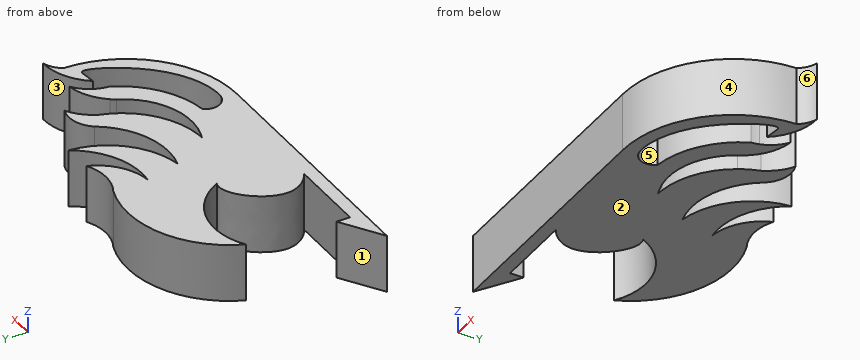
from build123d import *

# Parameters (mm, degrees)
F1_DEPTH = 25.4


with BuildPart() as f1:
    # F0 (on Top) → F1 (new body)
    with BuildSketch(Plane.XY):
        with BuildLine():
            add(Edge.make_bspline(
                [(-26.2610681984, -10.8273644), (-22.3250154222, -12.9399033802), (-6.7541943176, -14.1664240285), (-7.861061568, 17.5830890308), (-15.3270475566, 20.9516510367)],
                knots=[0.4911658302, 0.4911658302, 0.4911658302, 0.4911658302, 0.6402639099, 1, 1, 1, 1], degree=3))
            add(Edge.make_bspline(
                [(-15.3270475566, 20.9516510367), (-22.3564971203, 24.123253121), (-41.1418845104, 4.1977350509), (-30.2859655215, -8.6671412095), (-26.2610681984, -10.8273644)],
                knots=[0, 0, 0, 0, 0.3387023101, 0.4911658302, 0.4911658302, 0.4911658302, 0.4911658302], degree=3))
        make_face()
        with BuildLine():
            add(Edge.make_bspline(
                [(35.5182294418, -10.447258051), (31.9129186826, -10.220612291), (23.1955555043, -7.2820451281), (18.0529932429, 2.8715139484), (17.1729191086, 8.9899072036)],
                knots=[0.4660645619, 0.4660645619, 0.4660645619, 0.4660645619, 0.5346510085, 0.6442786993, 0.6442786993, 0.6442786993, 0.6442786993], degree=3))
            ThreePointArc((35.5182294418, -10.447258051), (30.0729748302, -6.5945561838), (31.0759395361, 0))
            ThreePointArc((31.0759395361, 0), (49.5151308357, 7.2590451113), (62.0112679899, 22.6390343159))
            ThreePointArc((62.0112679899, 22.6390343159), (62.2358256831, 24.395139963), (62.6415775007, 26.1184213282))
            add(Edge.make_bspline(
                [(54.4754700357, 26.7574300255), (57.3752815642, 26.5086516013), (60.1433747449, 26.2647226636), (62.6415775007, 26.1184213282)],
                knots=[0.9219128776, 0.9219128776, 0.9219128776, 0.9219128776, 0.9641346796, 0.9641346796, 0.9641346796, 0.9641346796], degree=3))
            ThreePointArc((54.4754700357, 26.7574300255), (53.7133787969, 25.7031684966), (53.0118979514, 24.6076434851))
            ThreePointArc((53.0118979514, 24.6076434851), (38.016967787, 10.0876095615), (17.1729191086, 8.9899072036))
        make_face()
        with BuildLine():
            ThreePointArc((-56.50515552, 32.3630547615), (-33.3182753375, 36.0316218628), (-15.3270475566, 20.9516510367))
            add(Edge.make_bspline(
                [(-26.2610681984, -10.8273644), (-22.3250154222, -12.9399033802), (-6.7541943176, -14.1664240285), (-7.861061568, 17.5830890308), (-15.3270475566, 20.9516510367)],
                knots=[0.4911658302, 0.4911658302, 0.4911658302, 0.4911658302, 0.6402639099, 1, 1, 1, 1], degree=3))
            Line((-26.2610681984, -10.8273644), (-60.464620338, -10.8273644))
            Line((-60.464620338, -10.8273644), (-60.464620338, -4.9215289764))
            Line((-60.464620338, -4.9215289764), (-78.4632340074, -16.4519678801))
            Line((-78.4632340074, -16.4519678801), (-14.9052012712, -16.4519678801))
            Line((-14.9052012712, -16.4519678801), (33.0445505679, -16.4519678801))
            ThreePointArc((33.0445505679, -16.4519678801), (67.0192612888, -2.5629170358), (81.5344079335, 31.1490573918))
            ThreePointArc((81.5344079335, 31.1490573918), (84.4106855525, 34.3353672495), (88.3062928915, 36.1380837858))
            ThreePointArc((88.3062928915, 36.1380837858), (77.0854781582, 33.5158631028), (68.3389529586, 26.0137952864))
            add(Edge.make_bspline(
                [(68.3389529586, 26.0137952864), (73.13500471, 26.2276507448), (80.3696253608, 30.0761350301), (65.6763095341, -1.3650666606), (43.6762193769, -10.9601053344), (35.5182294418, -10.447258051)],
                knots=[0, 0, 0, 0, 0.1043811632, 0.3108691907, 0.4660645619, 0.4660645619, 0.4660645619, 0.4660645619], degree=3))
            add(Edge.make_bspline(
                [(35.5182294418, -10.447258051), (31.9129186826, -10.220612291), (23.1955555043, -7.2820451281), (18.0529932429, 2.8715139484), (17.1729191086, 8.9899072036)],
                knots=[0.4660645619, 0.4660645619, 0.4660645619, 0.4660645619, 0.5346510085, 0.6442786993, 0.6442786993, 0.6442786993, 0.6442786993], degree=3))
            ThreePointArc((17.1729191086, 8.9899072036), (15.8161613784, 9.4543765839), (14.4833568484, 9.9836736917))
            ThreePointArc((14.4833568484, 9.9836736917), (15.7599932562, 10.0425488454), (17.0336540583, 10.1476914274))
            add(Edge.make_bspline(
                [(17.0336540583, 10.1476914274), (16.5524367293, 15.1345962527), (19.2361600934, 26.9166935874), (34.5605586177, 27.9160004318), (43.9602541666, 27.5027224979)],
                knots=[0.6512070875, 0.6512070875, 0.6512070875, 0.6512070875, 0.7409649976, 0.872432959, 0.872432959, 0.872432959, 0.872432959], degree=3))
            ThreePointArc((43.9602541666, 27.5027224979), (45.9259805238, 31.4321090753), (47.3872944713, 35.5756245553))
            ThreePointArc((47.3872944713, 35.5756245553), (51.1063153143, 41.2109006624), (56.3866607845, 45.4186797142))
            ThreePointArc((56.3866607845, 45.4186797142), (48.2264153253, 45.809802792), (41.481461376, 41.2002280354))
            ThreePointArc((41.481461376, 41.2002280354), (25.0576689955, 27.6740129875), (3.7966074888, 26.8574878573))
            ThreePointArc((3.7966074888, 26.8574878573), (23.5274065425, 37.3289516325), (32.4820913374, 57.7928125858))
            ThreePointArc((32.4820913374, 57.7928125858), (18.6619239349, 44.9253049217), (0, 42.0439206064))
            ThreePointArc((0, 42.0439206064), (12.1179065959, 46.7589869992), (19.8267325759, 57.2303533554))
            ThreePointArc((19.8267325759, 57.2303533554), (9.9133662879, 54.6642939776), (0, 57.2303533554))
            ThreePointArc((0, 57.2303533554), (-33.2620682112, 56.1796066262), (-56.50515552, 32.3630547615))
        make_face()
        with BuildLine():
            ThreePointArc((17.0336540583, 10.1476914274), (32.5838091219, 15.5874190212), (43.9602541666, 27.5027224979))
            add(Edge.make_bspline(
                [(17.0336540583, 10.1476914274), (16.5524367293, 15.1345962527), (19.2361600934, 26.9166935874), (34.5605586177, 27.9160004318), (43.9602541666, 27.5027224979)],
                knots=[0.6512070875, 0.6512070875, 0.6512070875, 0.6512070875, 0.7409649976, 0.872432959, 0.872432959, 0.872432959, 0.872432959], degree=3))
        make_face()
        with BuildLine():
            add(Edge.make_bspline(
                [(54.4754700357, 26.7574300255), (57.3752815642, 26.5086516013), (60.1433747449, 26.2647226636), (62.6415775007, 26.1184213282)],
                knots=[0.9219128776, 0.9219128776, 0.9219128776, 0.9219128776, 0.9641346796, 0.9641346796, 0.9641346796, 0.9641346796], degree=3))
            ThreePointArc((62.6415775007, 26.1184213282), (65.2892454144, 31.4686261622), (69.6213813016, 35.5756245553))
            ThreePointArc((69.6213813016, 35.5756245553), (61.1788209316, 32.6601387253), (54.4754700357, 26.7574300255))
        make_face()
    extrude(amount=F1_DEPTH)


solid = f1.part
Verification items for the finished model (mm, model axes). Face numbers are marked on the shaded views. A direction names the side the tool comes from. Coordinates: 2 decimals unless noted, no trailing zeros. Write each loop counter-clockwise with the first axis right and the second up, starting at its lowest first coordinate (ties: lowest second). Pieces come first, ordered by that corner, then holes. Notation, with made-up numbers: (85.25, 77.5) -> (103.25, 77.5) arc R20 ccw to (103.25, 96.5) -> close; hole circle Ø7 at (82, 12). An arc over 180 degrees is marked (long way). One line per item, written item: value. Start each with the question number.
Q1. Cross-section at C-C on y = 15. State how many separate pieces and enclosed holes the cut face has, and give its area (3 significant figures).
Q2. Access from +Z, -Z, +X, -X, +Y, -Y to the whole of each face (thin tool, end or side, straight path). Record for the marked faces 5 and 6.
Q3. Cross-section at B-B on y = 39. Enter the section's corners in (x, z), and give its area (3 significant figures).
Q4. Cross-section at A-A on y = 29. Enter the section's corners in (x, z), and give its area (3 significant figures).
Q5. Go/stop test with flat-tipped pins: P1, Ø1.5, axis at x = 34, z = 17, coming from the +Y side; P2, Ø2, axis at x = -42.5, y = 34.5, coming from the +Z side; P3, Ø1, axis at x = 71, y = 4.5, coming from the -Z side; P4, Ø4, axis at y = 45.5, z = 6, coming from the +X side. Record where each tip stops, or that it passes through.
Q6. Cross-section at D-D on y = 51. Enter the section's corners in (x, z).
Q7. Mould release check, pull along X, two halves, no side actions. Record for the marked faces 1, 2, 3 and 4: pulls with the +X half, pulls with the -X half, needs draft (parallel to the pull), parting line crosses it, or undercut.
Q8. Thickness scan on L1, parallel to Y at x = -31, z = 17; L2, parallel to Y at x = 22, z = 9; L3, parallel to X at y = 13.5, z = 23. Record the ranges inside material, lowest first. Write a range as from..to.
Checked values:
1. separate pieces: 3
1. enclosed holes: 0
1. area: 1,980 mm²
2. face 5: +Z, -Z
2. face 6: +Z, -Z, +X, -Y
3. outline: (-53.1, 0) -> (24.98, 0) -> (24.98, 25.4) -> (-53.1, 25.4) -> close; (39.99, 0) -> (49.34, 0) -> (49.34, 25.4) -> (39.99, 25.4) -> close
3. area: 2,220 mm²
4. outline: (-21.09, 0) -> (11.51, 0) -> (11.51, 25.4) -> (-21.09, 25.4) -> close; (28.08, 0) -> (44.78, 0) -> (44.78, 25.4) -> (28.08, 25.4) -> close; (56.44, 0) -> (63.77, 0) -> (63.77, 25.4) -> (56.44, 25.4) -> close; (70.87, 0) -> (81.45, 0) -> (81.45, 25.4) -> (70.87, 25.4) -> close
4. area: 1,710 mm²
5. P1: stops at y = 33.4
5. P2: passes through
5. P3: stops at z = 0
5. P4: stops at x = 56.39
6. outline: (-42.1, 0) -> (16.38, 0) -> (16.38, 25.4) -> (-42.1, 25.4) -> close; (27.25, 0) -> (31.25, 0) -> (31.25, 25.4) -> (27.25, 25.4) -> close
7. face 1: pulls with the -X half
7. face 2: needs draft
7. face 3: undercut
7. face 4: pulls with the +X half
8. L1: y = -16.45..-10.83, -7.02..11.34, 35.28..57.1
8. L2: y = -16.45..7.9, 11.01..26.68, 35.78..46.8
8. L3: x = -29.52..28.87, 43.9..56.22, 71.42..77.86
